```python
from build123d import *

# Parameters (mm, degrees)
F0_W     = 77.923713997
F0_H     = 109.7831092775
F1_DEPTH = 2


with BuildPart() as f1:
    # F0 (on Top) → F1 (new body)
    with BuildSketch(Plane.XY):
        Polygon((-98.5241234303, 94.8422709107), (-98.5241234303, 54.8422709107), (23.5521625727, 54.8422709107), (23.5521625727, 55.5602938927), align=None)
        Polygon((23.5521625727, 54.8422709107), (-98.5241234303, 54.8422709107), (-98.5241234303, -54.8019595444), (-98.5241234303, -54.9408383667), (23.5521625727, -54.9408383667), align=None)
        with Locations((62.5140195712, -0.049283728)):
            Rectangle(F0_W, F0_H)
        Polygon((23.5521625727, -55.2528910339), (23.5521625727, -54.9408383667), (-98.5241234303, -54.9408383667), (-98.5241234303, -94.7827324271), align=None)
    extrude(amount=F1_DEPTH)


solid = f1.part
```
Design review of the part built by this model. Coordinates are the model's own, in mm. Coordinates: 2 decimals unless noted, no trailing zeros. Write each loop counter-clockwise with the first axis right and the second up, starting at its lowest first coordinate (ties: lowest second). Pieces come first, ordered by that corner, then holes.
1) Add section C-C (y = -73). Write out the cut boundary in (x, z).
2) Insertion check: pin 1 (1 mm diameter, centred on x = 64.5, z = 1.5, fed in from +Y). The pin has a flat end and moves straight along its axis. Give the tip position at first contact, or say it passes through.
3) To check wall thickness, follow L1, parallel to Y at x = 44.5, z = 1.8; L2, parallel to Y at x = -12, z = 0.7. State the ranges of each line that lie inside material, in increasing order.
4) Add section B-B (x = 38). Write out the cut boundary in (y, z), plus the area to 3 significant figures.
5) Add section A-A (z = 1). Write out the cut boundary in (x, y).
Check result:
1. outline: (-98.52, 0) - (-31.25, 0) - (-31.25, 2) - (-98.52, 2) - close
2. pin 1: stops at y = 54.84
3. L1: y = -54.94 to 54.84
3. L2: y = -66.77 to 67
4. outline: (-54.94, 0) - (54.84, 0) - (54.84, 2) - (-54.94, 2) - close
4. area: 220 mm2
5. outline: (-98.52, -94.78) - (23.55, -55.25) - (23.55, -54.94) - (101.48, -54.94) - (101.48, 54.84) - (23.55, 54.84) - (23.55, 55.56) - (-98.52, 94.84) - close
